from build123d import *

# Parameters (mm, degrees)
REVOLVE1_ANGLE = 120


with BuildPart() as part:
    # Sketch1 → Revolve1 (revolve)
    with BuildSketch(Plane(origin=(0, 0, 0), x_dir=(1, 0, 0), z_dir=(0, 1, 0))):
        Polygon((0, -41.275), (0, 0), (-20.7, 0), (-20.7, -5), (-170.7, -27.5), (-520.7, -27.5), (-596.9, -27.5), (-596.9, 0), (-609.6, 0), (-609.6, -41.275), align=None)
        with BuildLine():
            Line((-596.9, -27.5), (-520.7, -27.5))
            add(Edge.make_bspline(
                [(-520.7, -27.5), (-596.9, -27.5), (-596.9, 0)],
                knots=[0, 0, 0, 1, 1, 1], degree=2))
            Line((-596.9, 0), (-596.9, -27.5))
        make_face()
    revolve(axis=Axis((0, 0, 0), (-1, 0, 0)), revolution_arc=REVOLVE1_ANGLE)


solid = part.part
Source: CAD feature listing. Evaluate the final solid. Frame: model axes, mm. A direction names the side the tool comes from. Round coordinates to 2 decimals unless told otherwise and drop trailing zeros. Write each loop counter-clockwise with the first axis right and the second up, starting at its lowest first coordinate (ties: lowest second). Pieces come first, ordered by that corner, then holes. Notation, with made-up numbers: M 4,76.5 L 11,76.5 A19 ccw 11,84.5 Z; hole C -38,34.5 d10. An arc over 180 degrees is marked long. One line per item, written item: value. Start each with the question number.
Item 1: Ray query, L1, parallel to Y at x = -425, z = -1.5; L2, parallel to Y at x = -394, z = 0.5; L3, parallel to Z at x = -132, y = 8.5. Return the intervals inside material, ascending. Write a range as from..to.
Item 2: Section query A-A (z = 33). Return the cut outline in (x, y), plus the area to 3 significant figures.
Item 3: Pin query (flat end, axial travel): pin 1 (3 mm diameter, centred on x = -270, y = 27.5, fed in from -Z); pin 2 (1 mm diameter, centred on x = -128, y = 27, fed in from -Z); pin 3 (10 mm diameter, centred on x = -186.5, z = 15, fed in from +Y). Return the tip coordinate at first contact, or that it passes through.
Item 4: Set-up query: faces 1 (the cylindrical face through (-348.15, 23.61, 14.1)), 2 (the flat face through (-609.6, 21, 11)). Return all of +Z, -Z, +X, -X, +Y, -Y with unobstructed straight access to the full face (end or side cutting, diameter ignored); none if empty.
Result set:
1. L1: y = 27.46..41.25
1. L2: y = 27.5..41.27
1. L3: z = 19.96..40.39
2. outline: M -609.6,0 L 0,0 L 0,24.79 L -609.6,24.79 Z
2. area: 15,100 mm²
3. pin 1: stops at z = -16.74
3. pin 2: stops at z = -15.88
3. pin 3: stops at y = 40.05
4. face 1: -Y
4. face 2: +Z, -Z, -X, +Y, -Y
